Geometry check sheet. Reference: the model listing, model coordinates, mm. Face numbers are marked on the shaded views. Coordinates: 2 decimals unless noted, no trailing zeros. Write each loop counter-clockwise with the first axis right and the second up, starting at its lowest first coordinate (ties: lowest second). Pieces come first, ordered by that corner, then holes. Notation, with made-up numbers: (27.25, 59.5) -> (73.25, 59.5) arc R17 cw to (73.25, 84.5) -> close; hole circle Ø2 at (36, 12). An arc over 180 degrees is marked (long way). One line per question, with ' | ' between items.
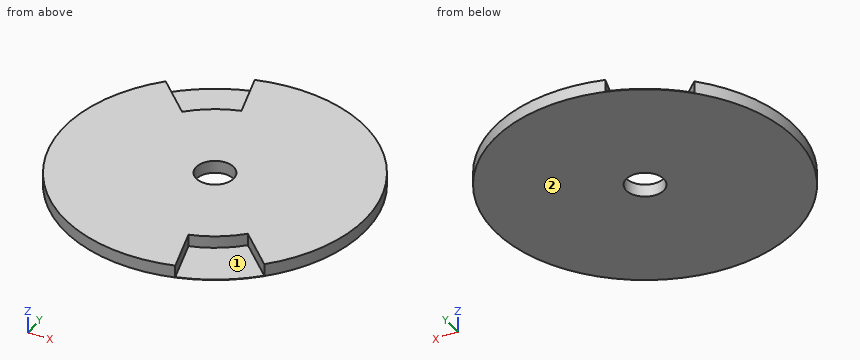
from build123d import *

# Parameters (mm, degrees)
SKETCH1_R          = 19.05
EXTRUDE1_DEPTH     = 1.5875
SKETCH2_R          = 2.38125
CUT_EXTRUDE1_DEPTH = 3.175
CUT_EXTRUDE2_DEPTH = 1.524


with BuildPart() as part:
    # Sketch1 → Extrude1 (new body)
    with BuildSketch(Plane.XY):
        Circle(SKETCH1_R)
    extrude(amount=EXTRUDE1_DEPTH)

    # Sketch2 → Cut-Extrude1 (cut)
    with BuildSketch(Plane.XY.offset(1.5875)):
        Circle(SKETCH2_R)
    extrude(amount=-CUT_EXTRUDE1_DEPTH, mode=Mode.SUBTRACT)

    # Sketch3 → Cut-Extrude2 (cut)
    with BuildSketch(Plane.XY.offset(1.5875)):
        with BuildLine():
            ThreePointArc((-4.930502809, 18.400886991), (-9.525, 16.497783942), (-13.470384182, 13.470384182))
            Line((-13.470384182, 13.470384182), (-8.980256121, 8.980256121))
            ThreePointArc((-8.980256121, 8.980256121), (-6.35, 10.998522628), (-3.287001873, 12.267257994))
            Line((-3.287001873, 12.267257994), (-4.930502809, 18.400886991))
        make_face()
        with BuildLine():
            Line((3.287001873, -12.267257994), (4.930502809, -18.400886991))
            ThreePointArc((4.930502809, -18.400886991), (9.525, -16.497783942), (13.470384182, -13.470384182))
            Line((13.470384182, -13.470384182), (8.980256121, -8.980256121))
            ThreePointArc((8.980256121, -8.980256121), (6.35, -10.998522628), (3.287001873, -12.267257994))
        make_face()
    extrude(amount=-CUT_EXTRUDE2_DEPTH, mode=Mode.SUBTRACT)


solid = part.part
1. Cross-section at A-A on y = 0. Record the boundary of the cut face in (x, z).
Worked answers:
outline: (-19.05, 0) -> (-2.38, 0) -> (-2.38, 1.59) -> (-19.05, 1.59) -> close; (2.38, 0) -> (19.05, 0) -> (19.05, 1.59) -> (2.38, 1.59) -> close
2. Material ranges on line 1 (Y direction, x = 0, z = 1); line 2 (X direction, y = 13, z = 0.5); line 3 (Y direction, x = -1.5, z = 0.2), recorded low to high. Write a range as from..to.
Worked answers:
line 1: -19.05..-2.38, 2.38..19.05 | line 2: -13.92..-13, -3.48..13.92 | line 3: -18.99..-1.85, 1.85..18.99
3. Cross-section at C-C on z = 1.1. Record the boundary of the cut face in (x, y).
Worked answers:
outline: (-13.47, 13.47) arc R19.05 ccw to (4.93, -18.4) -> (3.29, -12.27) arc R12.7 ccw to (8.98, -8.98) -> (13.47, -13.47) arc R19.05 ccw to (-4.93, 18.4) -> (-3.29, 12.27) arc R12.7 ccw to (-8.98, 8.98) -> close; hole circle Ø4.76 at (0, 0)
4. Go/stop test with flat-tipped pins: P1, Ø10.5, axis at x = 7.5, y = -14, coming from the +Z side; P2, Ø3, axis at x = -8, y = 12.5, coming from the +Z side. Record where each tip stops, or that it passes through.
Worked answers:
P1: z = 1.59 | P2: z = 0.06
5. Mould release check, pull along X, two halves, no side actions. Record for the marked faces 1 and 2: released by +X, released by -X, zero draft, split by the parting line, or undercut.
Worked answers:
face 1: undercut | face 2: zero draft
6. Cross-section at D-D on x = 4. Record the boundary of the cut face in (y, z), and give its area (3 significant figures).
Worked answers:
outline: (-18.63, 0) -> (18.63, 0) -> (18.63, 1.59) -> (-12.05, 1.59) -> (-12.05, 0.06) -> (-14.93, 0.06) -> (-14.93, 1.59) -> (-18.63, 1.59) -> close | area: 54.8 mm²
